Check sheet for the drawn part. Datum: minimum x, y, z corner. Units: mm. A direction names the side the tool comes from. Give positions to 0.01 mm unless a question says otherwise; leave off trailing zeros. Loops run counter-clockwise (first coordinate to the right, second up) from the corner with the lowest first, then second, coordinate; pieces in that order, holes last. Notation, with made-up numbers: (36, 77) - (62, 77) arc R26 cw to (62, 107) - close; hole circle Ø11 at (59.5, 89.25). An arc over 180 degrees is marked (long way). Answer in a Markdown table with one row per item.
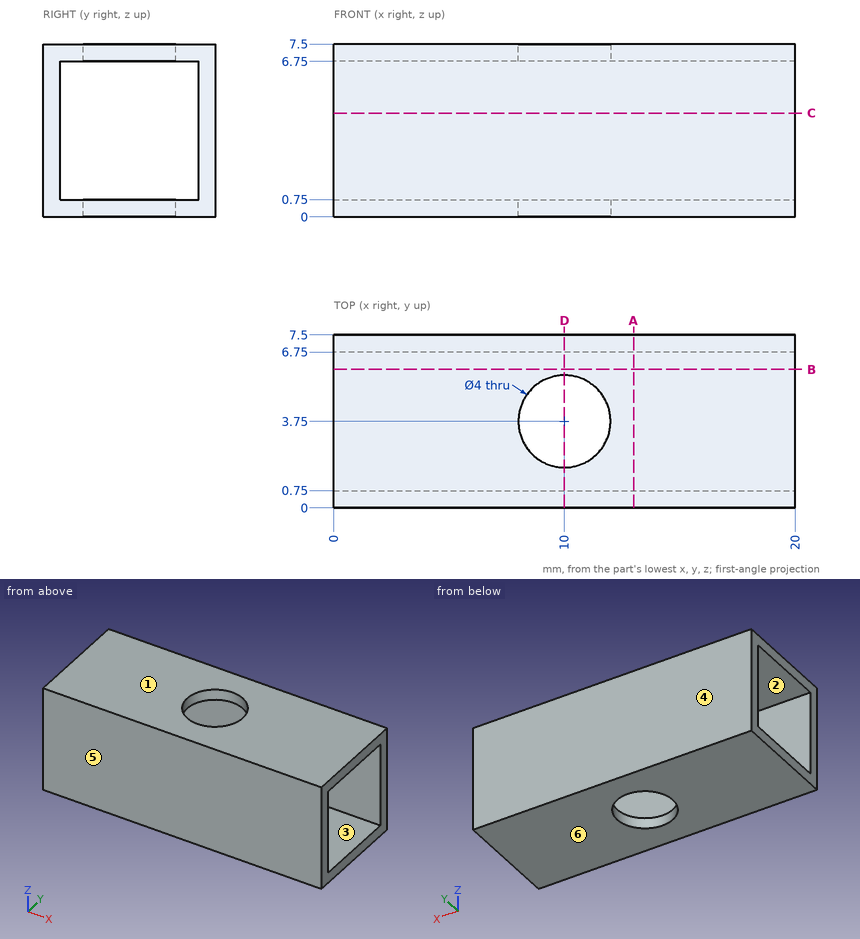
Q1. Thickness scan on line 1 (Z direction, x = 2.75, y = 3.25); line 2 (Y direction, x = 10, z = 7.15). Record the ranges inside material, lowest first.
Completed:
| item | result |
|---|---|
| line 1 | 0 to 0.75, 6.75 to 7.5 |
| line 2 | 0 to 1.75, 5.75 to 7.5 |
Q2. Sectioned sample at A-A (x = 13). Record the cut outline in (y, z).
Completed:
| item | result |
|---|---|
| outline | (0, 0) - (7.5, 0) - (7.5, 7.5) - (0, 7.5) - close; hole (0.75, 0.75) - (6.75, 0.75) - (6.75, 6.75) - (0.75, 6.75) - close |
Q3. Sectioned sample at B-B (y = 6). Record the cut outline in (x, z), and give its area (3 significant figures).
Completed:
| item | result |
|---|---|
| outline | (0, 0) - (20, 0) - (20, 0.75) - (0, 0.75) - close; (0, 6.75) - (20, 6.75) - (20, 7.5) - (0, 7.5) - close |
| area | 30.0 mm^2 |
Q4. Sectioned sample at D-D (x = 10). Record the cut outline in (y, z), and give its area (4 significant figures).
Completed:
| item | result |
|---|---|
| outline | (0, 0) - (1.75, 0) - (1.75, 0.75) - (0.75, 0.75) - (0.75, 6.75) - (1.75, 6.75) - (1.75, 7.5) - (0, 7.5) - close; (5.75, 0) - (7.5, 0) - (7.5, 7.5) - (5.75, 7.5) - (5.75, 6.75) - (6.75, 6.75) - (6.75, 0.75) - (5.75, 0.75) - close |
| area | 14.25 mm^2 |
Q5. Draft check along Y on the marked faces 3, 4, 5 and 6. Enter one of: +Y half, -Y half, draft (parallel to the pull), parting line (faces both ways), or undercut.
Completed:
| item | result |
|---|---|
| face 3 | undercut |
| face 4 | +Y half |
| face 5 | -Y half |
| face 6 | draft |
Q6. Tool access check on the marked faces 1 and 2. Record the directions out of +Z, -Z, +X, -X, +Y, -Y that give a thin tool (end or side, any length) a straight path to the whole face; none if there is none.
Completed:
| item | result |
|---|---|
| face 1 | +Z, +X, -X, +Y, -Y |
| face 2 | +X, -X |
Q7. Go/stop test with a flat-tipped pin: P1, Ø2.5, axis at x = 10, y = 3.75, coming from the -Z side. Record where the tip stops, or that it passes through.
Completed:
| item | result |
|---|---|
| P1 | through |
